```python
from build123d import *

# Parameters (mm, degrees)
CYLINDER860_R          = 1.5
CYLINDER860_DEPTH      = 60
CYLINDER859_R          = 1.5
CYLINDER859_DEPTH      = 60
BOX336_W               = 20
BOX336_H               = 40
BOX336_DEPTH           = 60
BOX336_PLACEMENT_ANGLE = 22
BOX410_W               = 20
BOX410_H               = 40
BOX410_DEPTH           = 60
BOX410_PLACEMENT_ANGLE = 22
BOX335_W               = 60
BOX335_H               = 40
BOX335_DEPTH           = 60
TUBE037_R              = 20.5
TUBE037_R_2            = 12
TUBE037_DEPTH          = 27
CUT469_PLACEMENT_ANGLE = 90


with BuildPart() as obj1:
    # Cylinder860 → Cylinder860 (new body)
    with BuildSketch(Plane(origin=(-3.5, 16, 0), x_dir=(1, 0, 0), z_dir=(0, 0, 1))):
        Circle(CYLINDER860_R)
    extrude(amount=CYLINDER860_DEPTH)


with BuildPart() as compound565:
    # Cylinder859 → Cylinder859 (new body)
    with BuildSketch(Plane(origin=(3.5, 16, 0), x_dir=(1, 0, 0), z_dir=(0, 0, 1))):
        Circle(CYLINDER859_R)
    extrude(amount=CYLINDER859_DEPTH)

    # Compound565: union obj1
    add(obj1.part)


with BuildPart() as krychle336:
    # Box336 → Box336 (new body)
    with BuildSketch(Plane.XY):
        with Locations((10, 20)):
            Rectangle(BOX336_W, BOX336_H)
    extrude(amount=BOX336_DEPTH)


with BuildPart() as krychle336_1:
    # Box336 placement: moved
    add(krychle336.part.rotate(Axis((0, 0, 0), (0, 0, -1)), BOX336_PLACEMENT_ANGLE))


with BuildPart() as krychle410:
    # Box410 → Box410 (new body)
    with BuildSketch(Plane.XY):
        with Locations((10, 20)):
            Rectangle(BOX410_W, BOX410_H)
    extrude(amount=BOX410_DEPTH)


with BuildPart() as krychle410_1:
    # Box410 placement: moved
    add(krychle410.part.moved(Location((-19.32, -5.18, 0))).rotate(Axis((-19.32, -5.18, 0), (0, 0, 1)), BOX410_PLACEMENT_ANGLE))


with BuildPart() as krychle335:
    # Box335 → Box335 (new body)
    with BuildSketch(Plane(origin=(-30, -35, 0), x_dir=(1, 0, 0), z_dir=(0, 0, 1))):
        with Locations((30, 20)):
            Rectangle(BOX335_W, BOX335_H)
    extrude(amount=BOX335_DEPTH)


with BuildPart() as cut469:
    # Tube037 → Tube037 (new body)
    with BuildSketch(Plane.XY.offset(23)):
        Circle(TUBE037_R)
        Circle(TUBE037_R_2, mode=Mode.SUBTRACT)
    extrude(amount=TUBE037_DEPTH)

    # Cut355: cut Krychle335
    add(krychle335.part, mode=Mode.SUBTRACT)

    # Cut357: cut Krychle410
    add(krychle410_1.part, mode=Mode.SUBTRACT)

    # Cut358: cut Krychle336
    add(krychle336_1.part, mode=Mode.SUBTRACT)

    # Cut469: cut Compound565
    add(compound565.part, mode=Mode.SUBTRACT)


with BuildPart() as cut469_1:
    # Cut469 placement: moved
    add(cut469.part.rotate(Axis((0, 0, 0), (0, 0, 1)), CUT469_PLACEMENT_ANGLE))


solid = cut469_1.part
```
Can you work these out from the model? Positions are in its coordinate system, mm. Round coordinates to 2 decimals unless told otherwise and drop trailing zeros. Loops run counter-clockwise (first coordinate to the right, second up) from the corner with the lowest first, then second, coordinate; pieces in that order, holes last.
Item 1: Please list where these lines run through material, in increasing order: L1, parallel to Y at x = -15.25, z = 35.75; L2, parallel to Y at x = -14.75, z = 29.75; L3, parallel to X at y = 4.75, z = 43.75.
Item 2: Suppose I cut it at A-A, the plane x = -16. Write out the boundary of the cut face in (y, z).
Item 3: Will these pins go through, and if not, where does the flat tip stop? pin 1 Ø4 at (y, z) = (-4.5, 36.5) entering from +X; pin 2 Ø2.5 at (x, y) = (-16, -3.5) entering from +Z; pin 3 Ø3 at (x, z) = (-17, 39.5) entering from +Y.
Item 4: Suppose I cut it at D-D, the plane y = -3. Write out the boundary of the cut face in (x, z), then the cut area to 3 significant figures.
Item 5: Suppose I cut it at C-C, the plane z = 46.75. Write out the boundary of the cut face in (x, y).
Item 6: If we mould it in two halves opening along X, with no side actions, what happens to faces 1 (the flat face through (-15.012, 6.065, 36.311)), 2 (the cylindrical face through (-15.425, -2.114, 36.311)), 3 (the flat face through (-16, 0, 50))? For each: +X half, -X half, draft (parallel to the pull), parting line (faces both ways), or undercut.
Item 7: Suppose I cut it at B-B, the plane y = 3.5. Write out the boundary of the cut face in (x, z).
Reported:
1. L1: y = -6 to -4.8, -2.2 to 2.2, 4.8 to 6.16
1. L2: y = -5.8 to -4.33, -2.67 to 2.67, 4.33 to 5.96
1. L3: x = -19.94 to -16.83, -15.17 to -11.76
2. outline: (-6.31, 23) - (-5, 23) - (-5, 50) - (-6.31, 50) - close; (-2, 23) - (2, 23) - (2, 50) - (-2, 50) - close; (5, 23) - (6.46, 23) - (6.46, 50) - (5, 50) - close
3. pin 1: stops at x = -11.18
3. pin 2: passes through
3. pin 3: stops at y = 7.47
4. outline: (-20.28, 23) - (-17.41, 23) - (-17.41, 50) - (-20.28, 50) - close; (-14.59, 23) - (-11.62, 23) - (-11.62, 50) - (-14.59, 50) - close
4. area: 157 mm2
5. outline: (-19.06, -7.54) - (-11.18, -4.36) arc R12 cw to (-11.13, 4.5) - (-19.01, 7.68) arc R20.5 ccw to start; hole circle Ø3 at (-16, -3.5); hole circle Ø3 at (-16, 3.5)
6. face 1: +X half
6. face 2: undercut
6. face 3: draft
7. outline: (-20.2, 23) - (-17.5, 23) - (-17.5, 50) - (-20.2, 50) - close; (-14.5, 23) - (-11.48, 23) - (-11.48, 50) - (-14.5, 50) - close
